Work out the finished part from the listing and answer in its coordinate system (mm). A direction names the side the tool comes from. Coordinates: 2 decimals unless noted, no trailing zeros. Loops run counter-clockwise (first coordinate to the right, second up) from the corner with the lowest first, then second, coordinate; pieces in that order, holes last.
```python
from build123d import *

# Parameters (mm, degrees)
F0_R     = 4
F1_DEPTH = 5
F3_DEPTH = 25


with BuildPart() as f1:
    # F0 (on Right) → F1 (new body)
    with BuildSketch(Plane.YZ):
        with BuildLine():
            Line((50, 15), (-61.757568, 15))
            Line((-61.757568, 15), (-61.757568, 12))
            Line((-61.757568, 12), (-81.757568, 12))
            Line((-81.757568, 12), (-15.860336, -11.984631))
            ThreePointArc((-15.860336, -11.984631), (-7.441737, -14.240388), (1.240672, -15))
            Line((1.240672, -15), (50, -15))
            ThreePointArc((50, -15), (65, 0), (50, 15))
        make_face()
        with Locations((35, 0)):
            Circle(F0_R, mode=Mode.SUBTRACT)
        with Locations((-5, 8)):
            Circle(F0_R, mode=Mode.SUBTRACT)
    extrude(amount=F1_DEPTH)

    # F2 (on face) → F3 (cut)
    with BuildSketch(Plane.YZ.offset(5)):
        with BuildLine():
            Line((-17.916537, 10), (-50.301027, 10))
            ThreePointArc((-50.301027, 10), (-52.270643, 8.347296), (-50.985068, 6.120615))
            Line((-50.985068, 6.120615), (-10.007906, -8.793852))
            ThreePointArc((-10.007906, -8.793852), (-9.597236, -8.938282), (-9.183521, -9.073739))
            ThreePointArc((-9.183521, -9.073739), (-7.004761, -8.396232), (-6.878676, -6.118051))
            Line((-6.878676, -6.118051), (-16.213294, 9.048315))
            ThreePointArc((-16.213294, 9.048315), (-16.940993, 9.745942), (-17.916537, 10))
        make_face()
        with BuildLine():
            Line((22.983953, 10), (6.245747, 10))
            ThreePointArc((6.245747, 10), (4.987106, 9.554292), (4.289451, 8.415823))
            Line((4.289451, 8.415823), (0.888546, -7.584177))
            ThreePointArc((0.888546, -7.584177), (1.29055, -9.258641), (2.844842, -10))
            Line((2.844842, -10), (24.864596, -10))
            ThreePointArc((24.864596, -10), (26.359077, -9.329108), (26.850922, -7.766527))
            Line((26.850922, -7.766527), (24.970279, 8.233473))
            ThreePointArc((24.970279, 8.233473), (24.31306, 9.494481), (22.983953, 10))
        make_face()
    extrude(amount=-F3_DEPTH, mode=Mode.SUBTRACT)


solid = f1.part
```
1. A cutting plane is placed at B-B, the plane y = 35. Give the vertices of the cut face in (x, z).
2. A cutting plane is placed at C-C, the plane z = -1.5. Give the vertices of the cut face in (x, y), then the cut area to 3 significant figures.
3. Each of these flat-tipped pins is pushed along its axis until it touches: P1, Ø9, axis at y = 35, z = 0, coming from the +X side; P2, Ø2.5, axis at x = 3, y = -68, coming from the +Z side; P3, Ø2.5, axis at x = 2.5, z = 13.5, coming from the -Y side; P4, Ø3, axis at x = 0.5, y = -14.5, coming from the -Z side. Where does it stop, or does it pass through?
4. A cutting plane is placed at A-A, the plane x = 3. Give the vertices of the cut face in (y, z), then the cut area to 3 significant figures.
5. A cutting plane is placed at D-D, the plane y = -5. Give the vertices of the cut face in (x, z).
6. Determine the mould class of faces 4 (the cylindrical face through (2, 65, 0)), 5 (the flat face through (2.535, -30.783, -1.232)), 6 (the flat face through (2.535, 25.924, 0.121)), 7 (the flat face through (5, 6.9, 10.2)) for opening direction Y: released by +Y, released by -Y, zero draft, split by the parting line, or undercut.
7. Straight lines are drawn through the part: probe 1 along Z at (x, y) = (3.3, 35); probe 2 along Z at (x, y) = (4.7, 6.5). For each, find the intervals that lie inside material, in ascending order.
8. For faces 1 (the flat face through (2, -61.758, 14)), 2 (the cylindrical face through (2.535, 1.275, -9.239)), 3 (the flat face through (2.465, -49.27, 0.176)), determine the directions among +Z, -Z, +X, -X, +Y, -Y from which every point of the face is accessible in a straight line to the end or side of a thin tool.
Answers below:
1. outline: (0, -15) - (5, -15) - (5, -4) - (0, -4) - close; (0, 4) - (5, 4) - (5, 15) - (0, 15) - close
2. outline: (0, -44.67) - (5, -44.67) - (5, -30.05) - (0, -30.05) - close; (0, -9.72) - (5, -9.72) - (5, 2.18) - (0, 2.18) - close; (0, 26.11) - (5, 26.11) - (5, 31.29) - (0, 31.29) - close; (0, 38.71) - (5, 38.71) - (5, 64.92) - (0, 64.92) - close
2. area: 290 mm2
3. P1: stops at x = 5
3. P2: stops at z = 12
3. P3: stops at y = -61.76
3. P4: stops at z = -12.93
4. outline: (-81.76, 12) - (-15.86, -11.98) arc R50 ccw to (1.24, -15) - (50, -15) arc R15 ccw to (50, 15) - (-61.76, 15) - (-61.76, 12) - close; hole (-50.99, 6.12) - (-10.01, -8.79) arc R20 ccw to (-9.18, -9.07) arc R2 ccw to (-6.88, -6.12) - (-16.21, 9.05) arc R2 ccw to (-17.92, 10) - (-50.3, 10) arc R2 ccw to start; hole circle Ø8 at (-5, 8); hole (0.89, -7.58) arc R2 ccw to (2.84, -10) - (24.86, -10) arc R2 ccw to (26.85, -7.77) - (24.97, 8.23) arc R2 ccw to (22.98, 10) - (6.25, 10) arc R2 ccw to (4.29, 8.42) - close; hole circle Ø8 at (35, 0)
4. area: 2,230 mm2
5. outline: (0, -14.61) - (5, -14.61) - (5, 4) - (0, 4) - close; (0, 12) - (5, 12) - (5, 15) - (0, 15) - close
6. face 4: released by +Y
6. face 5: undercut
6. face 6: undercut
6. face 7: zero draft
7. probe 1: z = -15 to -4, 4 to 15
7. probe 2: z = -15 to -10, 10 to 15
8. face 1: +Z, +X, -X, -Y
8. face 2: +X, -X
8. face 3: -Z, +X, -X, -Y
